from build123d import *

# Parameters (mm, degrees)
BOSS_EXTRUDE1_DEPTH      = 8.573703
BOSS_EXTRUDE1_DEPTH_BACK = 75.248703
SKETCH1_W                = 25.4
SKETCH1_H                = 25.4
SKETCH1_W_2              = 19.05
SKETCH1_H_2              = 19.05
SKETCH2_W                = 25.4
SKETCH2_H                = 25.4
SKETCH2_H_2              = 50.8
CUT_EXTRUDE1_DEPTH       = 365.478167069


with BuildPart() as part:
    # Sketch1 → Boss-Extrude1 (new, two sides: drawn at the far end of the back side and taken through both)
    with BuildSketch(Plane(origin=(115.396321255, 151.457671647, 0), x_dir=(-0.7954317200324988, 0.606043215262856, 0), z_dir=(-0.606043215262856, -0.7954317200324988, 0)).offset(-BOSS_EXTRUDE1_DEPTH_BACK)):
        with Locations((-209.448142065, -88.9)):
            Rectangle(SKETCH1_W, SKETCH1_H)
        with Locations((-209.448142065, -88.9)):
            Rectangle(SKETCH1_W_2, SKETCH1_H_2, mode=Mode.SUBTRACT)
    extrude(amount=BOSS_EXTRUDE1_DEPTH + BOSS_EXTRUDE1_DEPTH_BACK)

    # Sketch2 → Cut-Extrude1 (cut, through all)
    with BuildSketch(Plane.XY):
        with Locations((330.2, 79.375)):
            Rectangle(SKETCH2_W, SKETCH2_H)
        with Locations((279.4, 0)):
            Rectangle(SKETCH2_W, SKETCH2_H_2)
    extrude(amount=CUT_EXTRUDE1_DEPTH, mode=Mode.SUBTRACT)


solid = part.part
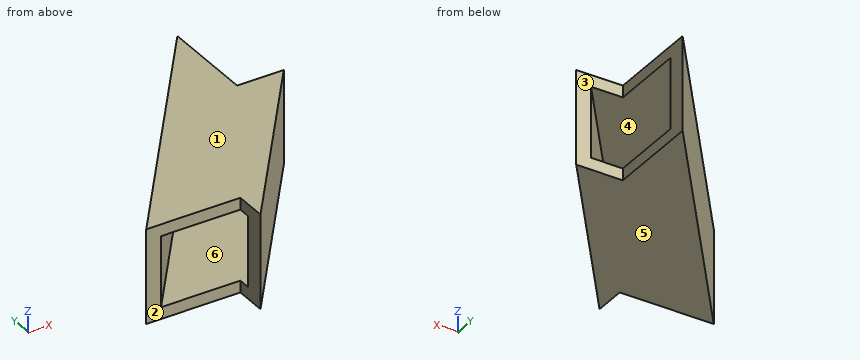
Read the model definition and answer for the solid it produces. Units are mm, in the model's axes. Face numbers are marked on the shaded views. A direction names the side the tool comes from. Coordinates: 2 decimals unless noted, no trailing zeros. Loops run counter-clockwise (first coordinate to the right, second up) from the corner with the lowest first, then second, coordinate; pieces in that order, holes last.
Q1. The part is cut by section D-D on x = 273. Write down the section's boundary in (y, z) (3 decimals), and give its area (3 significant figures).
Q2. Each of these flat-tipped pins is pushed along its axis until it touches: pin 1 Ø7.5 at (x, z) = (278.5, 90.5) entering from -Y; pin 2 Ø3 at (x, y) = (304, 76.5) entering from +Z; pin 3 Ø6.5 at (x, z) = (323, 84) entering from +Y (3 decimals); pin 4 Ø2.5 at (y, z) = (21, 83) entering from -X. Where does it stop, or does it pass through?
Q3. The mould has two halves that part along X. Classify the marked faces 5 and 6: +X half, -X half, draft (parallel to the pull), parting line (faces both ways), or undercut.
Q4. Which of the six approach directions +Z, -Z, +X, -X, +Y, -Y give full straight-line access (tool end or side, diameter ignored) to the marked faces 1, 2, 3 and 4?
Q5. The part is cut by section B-B on x = 307. Write down the section's boundary in (y, z) (3 decimals), and give its area (3 significant figures).
Q6. Consider probe 1 along Z at (x, y) = (287, 41) (3 decimals); probe 2 along Y at (x, z) = (315.5, 91.5); probe 3 along Y at (x, z) = (311, 98.25). Determine where each line is inside the solid, lowest interval first.
Q7. The part is cut by section A-A on z = 94.25. Write down the section's boundary in (x, y) (3 decimals), and give its area (3 significant figures).
Q8. The part is cut by section C-C on y = 54. Write down the section's boundary in (x, z) (3 decimals).
Results below:
1. outline: (25.4, 76.2) - (33.669, 76.2) - (33.669, 101.6) - (25.4, 101.6) - (25.4, 98.425) - (28.43, 98.425) - (28.43, 79.375) - (25.4, 79.375) - close
1. area: 152 mm2
2. pin 1: stops at y = 30.73
2. pin 2: stops at z = 101.6
2. pin 3: stops at y = 66.675
2. pin 4: stops at x = 292.1
3. face 5: draft
3. face 6: undercut
4. face 1: +Z, +X, -X, +Y, -Y
4. face 2: +Z, -Z, -X, -Y
4. face 3: +Z, -Z, +X, +Y
4. face 4: none
5. outline: (36.383, 76.2) - (78.294, 76.2) - (78.294, 101.6) - (36.383, 101.6) - close; hole (41.621, 79.375) - (73.055, 79.375) - (73.055, 98.425) - (41.621, 98.425) - close
5. area: 466 mm2
6. probe 1: z = 76.2 to 79.375, 98.425 to 101.6
6. probe 2: y = 47.54 to 52.78, 84.21 to 89.45
6. probe 3: y = 41.63 to 46.87, 78.3 to 83.54
7. outline: (266.7, 25.4) - (270.692, 25.4) - (317.5, 86.836) - (317.5, 92.075) - close; (292.1, 16.826) - (330.08, 66.675) - (326.088, 66.675) - (292.1, 22.065) - close
7. area: 444 mm2
8. outline: (288.49, 76.2) - (320.423, 76.2) - (320.423, 101.6) - (288.49, 101.6) - close; hole (292.482, 79.375) - (316.431, 79.375) - (316.431, 98.425) - (292.482, 98.425) - close
